```python
from build123d import *

# Parameters (mm, degrees)
F1_DEPTH = 101.6
F2_R     = 11.747271
F3_DEPTH = 101.6
F4_R     = 12.378993
F5_DEPTH = 101.6


with BuildPart() as f1:
    # F0 (on Front) → F1 (new body)
    with BuildSketch(Plane.XZ):
        Polygon((-18.419569, 4.604892), (-42.307448, 51.51723), (-63.892879, -50.366007), (68.209969, 9.49759), align=None)
    extrude(amount=F1_DEPTH)

    # F2 (on face) → F3 (join)
    with BuildSketch(Plane(origin=(0, 0, 0), x_dir=(-1, 0, 0), z_dir=(0, 1, 0))):
        with Locations((29.212283, -10.073202)):
            Circle(F2_R)
    extrude(amount=-F3_DEPTH)

    # F4 (on face) → F5 (cut)
    with BuildSketch(Plane(origin=(0, 0, 0), x_dir=(-1, 0, 0), z_dir=(0, 1, 0))):
        with Locations((29.500088, -9.49759)):
            Circle(F4_R)
    extrude(amount=-F5_DEPTH, mode=Mode.SUBTRACT)


solid = f1.part
```
Geometry: final body of the model. Coordinates: model frame, mm. A direction names the side the tool comes from. Round coordinates to 2 decimals unless told otherwise and drop trailing zeros. Order: outer loops, then holes, each group sorted by start corner. A loop starts at its lowest first (then second) coordinate and runs counter-clockwise, first axis right, second up. Notation, with made-up numbers: (60, 27.5) -> (71, 27.5) arc R8 cw to (71, 39.5) -> close; hole circle Ø5 at (69.5, 1). An arc over 180 degrees is marked (long way). Use CSV: the item, a comma, the result in double quotes. Start each with the question number.
1) First-contact query: pin 1 Ø6 at (x, y) = (39.5, -45.5) entering from -Z; pin 2 Ø3 at (y, z) = (-66, 34) entering from +X; pin 3 Ø2 at (x, y) = (43, -41.5) entering from +Z. Flat tips, straight axial feed; report the tip coordinate or a pass-through.
2) Material intervals for line 1 along X through (y, z) = (-53.5, -5.5); line 2 along X through (y, z) = (-67.5, -6); line 3 along Z through (x, y) = (14.5, -79), sorted ascending. Write a range as from..to.
3) Set-up query: faces 1 (the face through (-52.95, -50.09, 1.29)), 2 (the face through (25.502, -50.089, 7.085)). Return all of +Z, -Z, +X, -X, +Y, -Y with unobstructed straight access to the full face (end or side cutting, diameter ignored); none if empty.
4) Section C-C (y = -14). Return the cut outline in (x, z), and give its area (3 significant figures).
5) Section B-B (z = -13.5). Return the cut outline in (x, y).
6) Section A-A (x = -36). Return the cut outline in (y, z).
7) Draft query along Z for faces 3 (the face through (-18, -101.6, 1)), 4 (the face through (1.234, -50.089, -20.853)), 5 (the face through (-41.307, -50.089, -5.779)). Return one class per face: +Z half, -Z half, draft (parallel to the pull), parting line (faces both ways), or undercut.
8) Section D-D (x = 31). Return the cut outline in (y, z), and give its area (3 significant figures).
Returned:
1,pin 1,"stops at z = -4.87"
1,pin 2,"stops at x = -32.62"
1,pin 3,"stops at z = 8.13"
2,line 1,"x = -54.39..-41.22, -17.78..35.11"
2,line 2,"x = -54.49..-41.37, -17.63..34.01"
2,line 3,"z = -14.84..6.46"
3,face 1,"+Z, -X, +Y, -Y"
3,face 2,"+Z, +Y, -Y"
4,outline,"(-63.89, -50.37) -> (68.21, 9.5) -> (-18.42, 4.6) -> (-42.31, 51.52) -> close; hole circle Ø24.76 at (-29.5, -9.5)"
4,area,"3,510 mm²"
5,outline,"(-56.08, -101.6) -> (-41.21, -101.6) -> (-41.21, 0) -> (-56.08, 0) -> close; (-17.79, -101.6) -> (17.46, -101.6) -> (17.46, 0) -> (-17.79, 0) -> close"
6,outline,"(-101.6, -37.73) -> (0, -37.73) -> (0, -20.03) -> (-101.6, -20.03) -> close; (-101.6, 1.04) -> (0, 1.04) -> (0, 39.13) -> (-101.6, 39.13) -> close"
7,face 3,"draft"
7,face 4,"-Z half"
7,face 5,"undercut"
8,outline,"(-101.6, -7.36) -> (0, -7.36) -> (0, 7.4) -> (-101.6, 7.4) -> close"
8,area,"1,500 mm²"
